Design review of the part built by this model. Coordinates are the model's own, in mm. Face numbers are marked on the shaded views. A direction names the side the tool comes from. Coordinates: 2 decimals unless noted, no trailing zeros. Order: outer loops, then holes, each group sorted by start corner. A loop starts at its lowest first (then second) coordinate and runs counter-clockwise, first axis right, second up. Notation, with made-up numbers: (-19.75, 88.25) - (29.25, 88.25) arc R9 ccw to (29.25, 98.25) - close; hole circle Ø11 at (86.5, -17). An arc over 180 degrees is marked (long way). Write item = value, one per line. Start each with the question number.
```python
from build123d import *

# Parameters (mm, degrees)
CIRPATTERN1_COUNT = 2
CIRPATTERN1_ANGLE = 90


with BuildPart() as part:
    # BodySke → Base-Revolve (revolve)
    with BuildSketch(Plane.XY, mode=Mode.PRIVATE) as base_revolve_sk:
        with BuildLine():
            Line((2.032, 1.4224), (2.032, 2.7813))
            Line((2.032, 2.7813), (1.075646615, 2.7813))
            ThreePointArc((1.075646615, 2.7813), (0.960371669, 2.753635341), (0.87020729, 2.676667612))
            ThreePointArc((0.87020729, 2.676667612), (0.223015279, 1.407285528), (0, 0))
            Line((0, 0), (9.9695, 0))
            Line((9.9695, 0), (9.9695, 1.4224))
            Line((9.9695, 1.4224), (2.032, 1.4224))
        make_face()
    revolve(base_revolve_sk.sketch.rotate(Axis((-25.4, 0, 0), (1, 0, 0)), 90), axis=Axis((-25.4, 0, 0), (1, 0, 0)))

    # Sketch3 → Cut-Loft1 section 0
    with BuildSketch(Plane(origin=(0, 0, 0), x_dir=(0, 0, -1), z_dir=(1, 0, 0))):
        with BuildLine():
            Line((0.4064, -1.8161), (-0.4064, -1.8161))
            Line((-0.4064, -1.8161), (-0.4064, 1.8161))
            Line((-0.4064, 1.8161), (0.4064, 1.8161))
            Line((0.4064, 1.8161), (0.4064, -1.8161))
        make_face()
    # Sketch4 → Cut-Loft1 section 1
    with BuildSketch(Plane(origin=(2.0066, 0, 0), x_dir=(0, 0, -1), z_dir=(1, 0, 0))):
        with BuildLine():
            Line((0.2032, -0.2032), (-0.2032, -0.2032))
            Line((-0.2032, -0.2032), (-0.2032, 0.2032))
            Line((-0.2032, 0.2032), (0.2032, 0.2032))
            Line((0.2032, 0.2032), (0.2032, -0.2032))
        make_face()
    cut_loft1 = loft(mode=Mode.SUBTRACT)

    # CirPattern1: Cut-Loft1 ×2 about axis
    cirpattern1_axis = Axis((0, 0, 0), (1, 0, 0))
    for i in range(1, CIRPATTERN1_COUNT):
        add(cut_loft1.rotate(cirpattern1_axis, i * CIRPATTERN1_ANGLE / (CIRPATTERN1_COUNT - 1)), mode=Mode.SUBTRACT)


solid = part.part
```
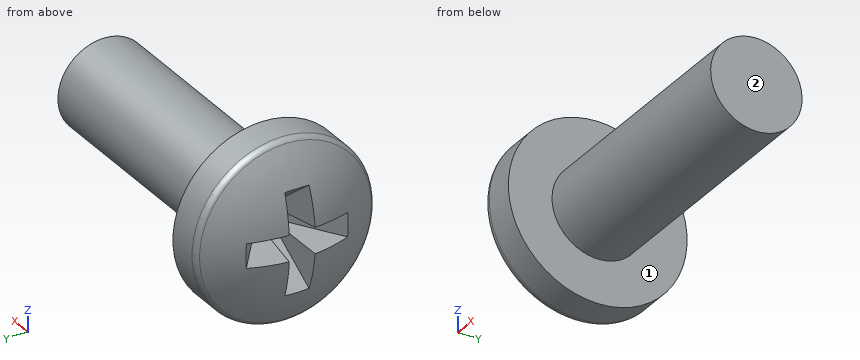
Item 1: For P1, Ø3, axis at x = 8, z = -0.5, coming from the +Y side; P2, Ø1.5, axis at y = 0, z = -1.5, coming from the -X side, all flat-tipped, find the tip position at first contact; note any pin that passes through.
Item 2: For line 1 (Y direction, x = 1, z = 0.55); line 2 (Y direction, x = 3.25, z = -0.05); line 3 (Z direction, x = 3.5, y = 1), list the stretches that pass through material, from the lowest coordinate up.
Item 3: For the marked faces 1 and 2, list the 3-axis set-ups (+Z, -Z, +X, -X, +Y, -Y) from which the entire face can be reached by the end or side of a thin tool; tool diameter is ignored.
Item 4: Add section A-A on x = 7.75. Give the boundary of the cut face in (y, z).
Worked out:
q1.P1 = 1.42
q1.P2 = 0.1
q2.line_1 = -2.71 to -0.31, 0.31 to 2.71
q2.line_2 = -1.42 to 1.42
q2.line_3 = -1.01 to 1.01
q3.face_1 = +X
q3.face_2 = +Z, -Z, +X, +Y, -Y
q4.outline = circle Ø2.84 at (0, 0)
